Check sheet for the drawn part. Datum: minimum x, y, z corner. Units: mm. A direction names the side the tool comes from. Coordinates: 2 decimals unless noted, no trailing zeros. Loops run counter-clockwise (first coordinate to the right, second up) from the corner with the lowest first, then second, coordinate; pieces in that order, holes last.
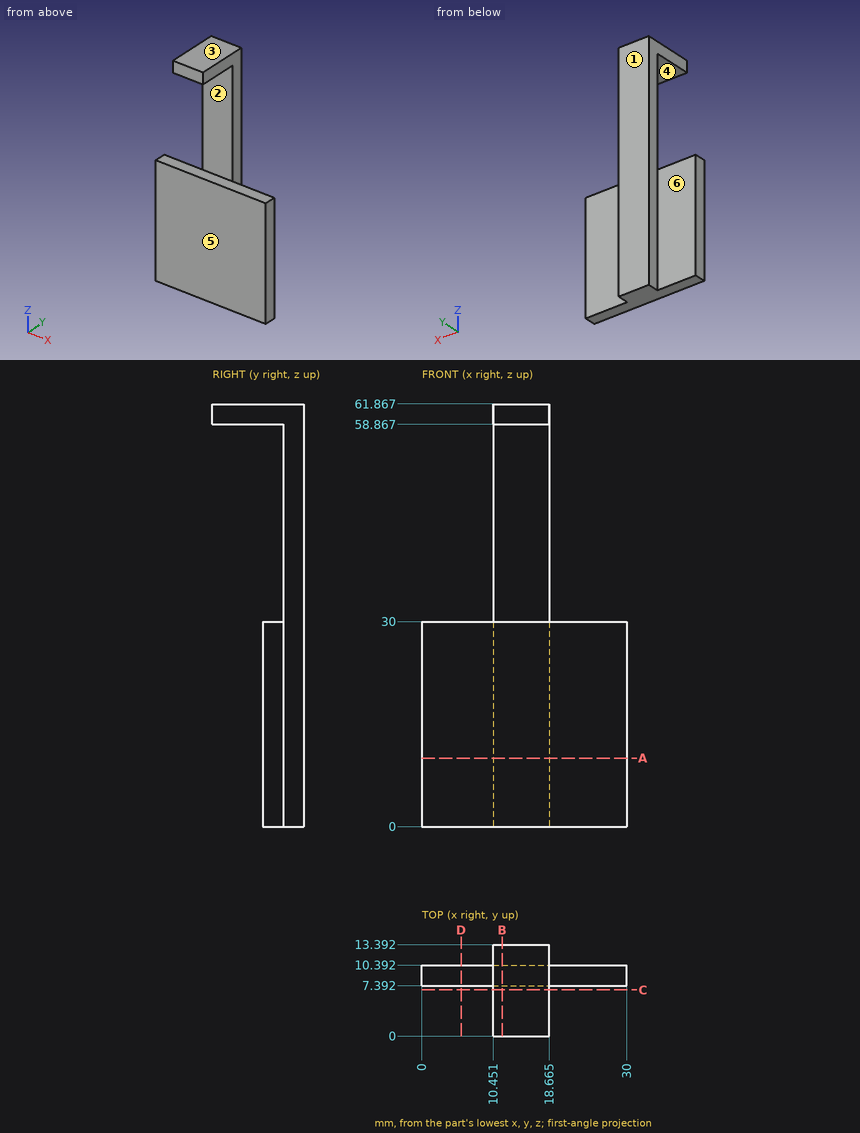
1) Scan lines: line 1 (Z direction, x = 16.25, y = 6.25); line 2 (Y direction, x = 11.25, z = 34); line 3 (X direction, y = 11, z = 51.5) (1 decimal). Record each from-to range of solid material in increasing order.
Answer sheet:
line 1: z = 58.87 to 61.87
line 2: y = 10.39 to 13.39
line 3: x = 10.5 to 18.7
2) Mould release check, pull along Z, two halves, no side actions. Record for the marked faces 1, 2 and 3: +Z half, -Z half, draft (parallel to the pull), parting line (faces both ways), or undercut.
Answer sheet:
face 1: draft
face 2: undercut
face 3: +Z half
3) Section check B-B on x = 11.75. Enter the section's corners in (y, z), plus the area to 3 significant figures.
Answer sheet:
outline: (0, 58.87) - (10.39, 58.87) - (10.39, 30) - (7.39, 30) - (7.39, 0) - (13.39, 0) - (13.39, 61.87) - (0, 61.87) - close
area: 307 mm2
4) Section check A-A on z = 10. Enter the section's corners in (x, y) (1 decimal).
Answer sheet:
outline: (0, 7.4) - (30, 7.4) - (30, 10.4) - (18.7, 10.4) - (18.7, 13.4) - (10.5, 13.4) - (10.5, 10.4) - (0, 10.4) - close
5) Section check D-D on x = 5.75. Enter the section's corners in (y, z).
Answer sheet:
outline: (7.39, 0) - (10.39, 0) - (10.39, 30) - (7.39, 30) - close
6) Depth check by flat-ended pin: pin 1 (5 mm diameter, centred on x = 11.5, z = 40.5, fed in from -Y); pin 2 (3 mm diameter, centred on x = 4.5, z = 6.5, fed in from -Y); pin 3 (8.5 mm diameter, centred on x = 4, z = 10, fed in from +Y); pin 4 (10 mm diameter, centred on x = 26.5, z = 39, fed in from -Y). Enter the tip coordinate at first touch or a pass-through.
Answer sheet:
pin 1: stops at y = 10.39
pin 2: stops at y = 7.39
pin 3: stops at y = 10.39
pin 4: passes through
7) Section check C-C on y = 6.75. Enter the section's corners in (x, z) (1 decimal).
Answer sheet:
outline: (10.5, 58.9) - (18.7, 58.9) - (18.7, 61.9) - (10.5, 61.9) - close
8) Set-up check for the marked faces 4, 5 and 6: record each of +Z, -Z, +X, -X, +Y, -Y from which the full face is reachable in a straight line by a thin tool's end or side.
Answer sheet:
face 4: +X, -X, -Y
face 5: -Z, +X, -X, -Y
face 6: +Z, -Z, -X, +Y
